from build123d import *

# Parameters (mm, degrees)
EXTRUDE_1_DEPTH = 1.26


with BuildPart() as part:
    # Model → 凸台-拉伸1 (new body)
    with BuildSketch(Plane.XY):
        with BuildLine():
            Line((490.799011507, 297.269554061), (490.799011507, 293.800954061))
            Line((490.799011507, 293.800954061), (490.799011507, 292.024354061))
            Line((490.799011507, 292.024354061), (490.622317978, 291.628783411))
            Line((490.622317978, 291.628783411), (490.291411507, 291.516754061))
            Line((490.291411507, 291.516754061), (489.487672027, 291.516754061))
            Line((489.487672027, 291.516754061), (489.281948064, 291.476958221))
            Line((489.281948064, 291.476958221), (489.149260696, 291.389854061))
            Line((489.149260696, 291.389854061), (489.046979347, 291.176662061))
            Line((489.046979347, 291.176662061), (489.022411507, 291.009154061))
            Line((489.022411507, 291.009154061), (489.022411507, 285.044854061))
            ThreePointArc((489.022411507, 285.044854061), (489.156337447, 284.700557005), (489.487711507, 284.537254061))
            Line((489.487711507, 284.537254061), (490.883611507, 284.537254061))
            Line((490.883611507, 284.537254061), (492.364111507, 286.017754061))
            Line((492.364111507, 286.017754061), (492.364111507, 287.117554061))
            Line((492.364111507, 287.117554061), (491.433481153, 287.117554061))
            Line((491.433481153, 287.117554061), (491.037940858, 287.29424759))
            Line((491.037940858, 287.29424759), (490.925911507, 287.625154061))
            Line((490.925911507, 287.625154061), (490.925911507, 287.921254061))
            Line((490.925911507, 287.921254061), (491.102605037, 288.31682471))
            Line((491.102605037, 288.31682471), (491.433511507, 288.428854061))
            Line((491.433511507, 288.428854061), (492.491011507, 288.428854061))
            Line((492.491011507, 288.428854061), (492.491011507, 290.374654061))
            Line((492.491011507, 290.374654061), (492.66027648, 290.75646672))
            Line((492.66027648, 290.75646672), (492.956311507, 290.882254061))
            Line((492.956311507, 290.882254061), (493.84460586, 290.882254061))
            Line((493.84460586, 290.882254061), (494.20148544, 291.05894759))
            Line((494.20148544, 291.05894759), (494.309911507, 291.389854061))
            Line((494.309911507, 291.389854061), (494.309911507, 296.000554061))
            Line((494.309911507, 296.000554061), (494.374646074, 296.245014221))
            Line((494.374646074, 296.245014221), (494.479015049, 296.381254061))
            Line((494.479015049, 296.381254061), (494.65360679, 296.483586221))
            Line((494.65360679, 296.483586221), (494.817511507, 296.508154061))
            Line((494.817511507, 296.508154061), (503.192882713, 296.508154061))
            Line((503.192882713, 296.508154061), (503.588482157, 296.331460531))
            Line((503.588482157, 296.331460531), (503.700511507, 296.000554061))
            Line((503.700511507, 296.000554061), (503.700511507, 291.389854061))
            Line((503.700511507, 291.389854061), (503.877205037, 290.994283411))
            Line((503.877205037, 290.994283411), (504.208111507, 290.882254061))
            Line((504.208111507, 290.882254061), (505.054032978, 290.882254061))
            Line((505.054032978, 290.882254061), (505.449682157, 290.688050362))
            Line((505.449682157, 290.688050362), (505.561711507, 290.374654061))
            Line((505.561711507, 290.374654061), (505.561711507, 288.428854061))
            Line((505.561711507, 288.428854061), (506.619129356, 288.428854061))
            Line((506.619129356, 288.428854061), (507.001024166, 288.252160531))
            Line((507.001024166, 288.252160531), (507.126811507, 287.921254061))
            Line((507.126811507, 287.921254061), (507.126811507, 287.625154061))
            Line((507.126811507, 287.625154061), (506.932607808, 287.229583411))
            Line((506.932607808, 287.229583411), (506.619211507, 287.117554061))
            Line((506.619211507, 287.117554061), (505.942411507, 287.117554061))
            Line((505.942411507, 287.117554061), (505.942411507, 286.525354055))
            ThreePointArc((505.942411507, 286.525354055), (506.549193576, 285.114196381), (507.972811507, 284.537254055))
            Line((507.972811507, 284.537254055), (508.522711502, 284.537254055))
            ThreePointArc((508.522711502, 284.537254055), (508.881638908, 284.685926655), (509.030311507, 285.044854061))
            Line((509.030311507, 285.044854061), (509.030311507, 291.009154061))
            Line((509.030311507, 291.009154061), (508.853617978, 291.40472471))
            Line((508.853617978, 291.40472471), (508.522711507, 291.516754061))
            Line((508.522711507, 291.516754061), (507.718966182, 291.516754061))
            Line((507.718966182, 291.516754061), (507.337198848, 291.69344759))
            Line((507.337198848, 291.69344759), (507.211411507, 292.024354061))
            Line((507.211411507, 292.024354061), (507.211411507, 299.046154061))
            Line((507.211411507, 299.046154061), (507.171615667, 299.56111223))
            Line((507.171615667, 299.56111223), (507.084511507, 299.934454061))
            Line((507.084511507, 299.934454061), (503.869711507, 310.382554061))
            ThreePointArc((503.869711507, 310.382554061), (502.775635028, 311.908062049), (500.993311507, 312.497554061))
            Line((500.993311507, 312.497554061), (497.017111507, 312.497554061))
            ThreePointArc((497.017111507, 312.497554061), (495.247553689, 311.912414538), (494.183011507, 310.382554061))
            Line((494.183011507, 310.382554061), (490.925864157, 299.934454061))
            Line((490.925864157, 299.934454061), (490.823579347, 299.450764051))
            Line((490.823579347, 299.450764051), (490.799011507, 299.046154061))
            Line((490.799011507, 299.046154061), (490.799011507, 297.269554061))
        make_face()
        with BuildLine():
            Line((499.005211507, 310.001854061), (499.893511507, 310.001854061))
            ThreePointArc((499.893511507, 310.001854061), (501.078970997, 309.62259882), (501.797011507, 308.605954061))
            Line((501.797011507, 308.605954061), (503.827347931, 302.091754061))
            Line((503.827347931, 302.091754061), (503.840525184, 301.061837722))
            Line((503.840525184, 301.061837722), (503.4889366, 300.315154061))
            Line((503.4889366, 300.315154061), (502.680170534, 299.676222374))
            Line((502.680170534, 299.676222374), (501.881611507, 299.511454061))
            Line((501.881611507, 299.511454061), (499.005211507, 299.511454061))
            Line((499.005211507, 299.511454061), (496.12871426, 299.511454061))
            Line((496.12871426, 299.511454061), (495.132361574, 299.775167827))
            Line((495.132361574, 299.775167827), (494.521372494, 300.315154061))
            Line((494.521372494, 300.315154061), (494.15297783, 301.28253408))
            Line((494.15297783, 301.28253408), (494.225311507, 302.091754061))
            Line((494.225311507, 302.091754061), (496.213411507, 308.605954061))
            ThreePointArc((496.213411507, 308.605954061), (496.961295967, 309.617562087), (498.159211507, 310.001854061))
            Line((498.159211507, 310.001854061), (499.005211507, 310.001854061))
        make_face(mode=Mode.SUBTRACT)
    extrude(amount=EXTRUDE_1_DEPTH)


solid = part.part
Geometry check sheet. Reference: the model listing, model coordinates, mm. A direction names the side the tool comes from. Give positions to 0.01 mm unless a question says otherwise; leave off trailing zeros. Write each loop counter-clockwise with the first axis right and the second up, starting at its lowest first coordinate (ties: lowest second). Pieces come first, ordered by that corner, then holes.
1) Thickness scan on line 1 (X direction, y = 307.5, z = 0.15); line 2 (Y direction, x = 497.25, z = 0.6); line 3 (X direction, y = 286.75, z = 0.15). Record the ranges inside material, lowest first.
Values follow:
line 1: x = 493.28 to 495.88, 502.14 to 504.76
line 2: y = 296.51 to 299.51, 309.79 to 312.5
line 3: x = 489.02 to 492.36, 505.94 to 509.03
2) Release check for a two-part mould opening along X. For faces 6 (the face through (509.03, 288, 1)), 7 (the face through (508, 291.517, 1)), 8 (the face through (494.19, 301.68, 0.62)) record: released by +X, released by -X, zero draft, split by the parting line, or undercut.
Values follow:
face 6: released by +X
face 7: zero draft
face 8: undercut
3) Cross-section at B-B (y = 289.25). Record the boundary of the cut face in (x, z).
Values follow:
outline: (489.02, 0) - (492.49, 0) - (492.49, 1.26) - (489.02, 1.26) - close; (505.56, 0) - (509.03, 0) - (509.03, 1.26) - (505.56, 1.26) - close
4) Cross-section at A-A (y = 294.75). Record the boundary of the cut face in (x, z).
Values follow:
outline: (490.8, 0) - (494.31, 0) - (494.31, 1.26) - (490.8, 1.26) - close; (503.7, 0) - (507.21, 0) - (507.21, 1.26) - (503.7, 1.26) - close
5) Cross-section at C-C (x = 504.5). Record the boundary of the cut face in (y, z), plus the area to 3 significant figures.
Values follow:
outline: (290.88, 0) - (308.33, 0) - (308.33, 1.26) - (290.88, 1.26) - close
area: 22.0 mm2
6) Go/stop test with flat-tipped pins: pin 1 Ø0.6 at (x, z) = (508, 1) entering from +Y; pin 2 Ø0.7 at (x, z) = (493.5, 0.5) entering from -Y; pin 3 Ø1.5 at (x, y) = (496.5, 296) entering from +Z; pin 4 Ø0.6 at (y, z) = (294, 1) entering from -X. Record where each tip stops, or that it passes through.
Values follow:
pin 1: stops at y = 291.53
pin 2: stops at y = 290.88
pin 3: stops at z = 1.26
pin 4: stops at x = 490.8
7) Set-up check for faces 1 (the face through (498, 299, 0)), 2 (the face through (506, 288.429, 1)), 3 (the face through (490.799, 296, 1)), 4 (the face through (506.534, 285.13, 0.621)), 5 (the face through (499, 312.498, 1)): record each of +Z, -Z, +X, -X, +Y, -Y from which the full face is reachable in a straight line by a thin tool's end or side.
Values follow:
face 1: -Z, +X, -X, +Y, -Y
face 2: +Z, -Z
face 3: +Z, -Z, -X, +Y
face 4: +Z, -Z, -Y
face 5: +Z, -Z, +X, -X, +Y
